Here's the drawing with two shaded views (mm, measured from the low corner). I have some questions. A direction names the side the tool comes from. Round coordinates to 2 decimals unless told otherwise and drop trailing zeros. Write each loop counter-clockwise with the first axis right and the second up, starting at its lowest first coordinate (ties: lowest second). Pieces come first, ordered by that corner, then holes. Notation, with made-up numbers: M -15,-7.75 L 39,-7.75 A33 ccw 39,24.25 Z; hole C 6,43 d4. An arc over 180 degrees is marked long. Answer as a JSON object with one key per item and string values. Group by question number.
1) If we mould it in two halves opening along Z, with no side actions, what happens to the marked faces 3, 4 and 5? For each: +Z half, -Z half, draft (parallel to the pull), parting line (faces both ways), or undercut.
2) On a 3-axis mill with a long thin cutter (end or side, diameter ignored), from which of +Z, -Z, +X, -X, +Y, -Y can I reach the whole of each face in a straight line? I mean the marked faces 1 and 2. Say none if no direction works.
3) I'm going to push flat-ended pins straight in: pin 1 Ø5 at (y, z) = (20.5, 49.5) entering from +X; pin 2 Ø3 at (y, z) = (24.5, 70) entering from -X; pin 3 Ø5 at (x, y) = (79, 24) entering from +Z; pin 4 Ø3 at (x, y) = (111.5, 23) entering from -Z. Where does each tip first touch, or does it pass through?
4) Suppose I cut it at B-B, the plane z = 58. Write out the boundary of the cut face in (x, y), and give its area (3 significant figures).
5) Please list where these lines run through material, in increasing order: L1, parallel to X at y = 27, z = 58; L2, parallel to Z at x = 142, y = 17; L3, parallel to Y at x = 118.5, z = 93. Write a range as [from, to].
6) Suppose I cut it at A-A, the plane x = 113. Write out the boundary of the cut face in (y, z).
7) Suppose I cut it at C-C, the plane x = 90.5. Write out the boundary of the cut face in (y, z), and give its area (3 significant figures).
8) Suppose I cut it at D-D, the plane z = 30. Write out the boundary of the cut face in (x, y), and give its area (3 significant figures).
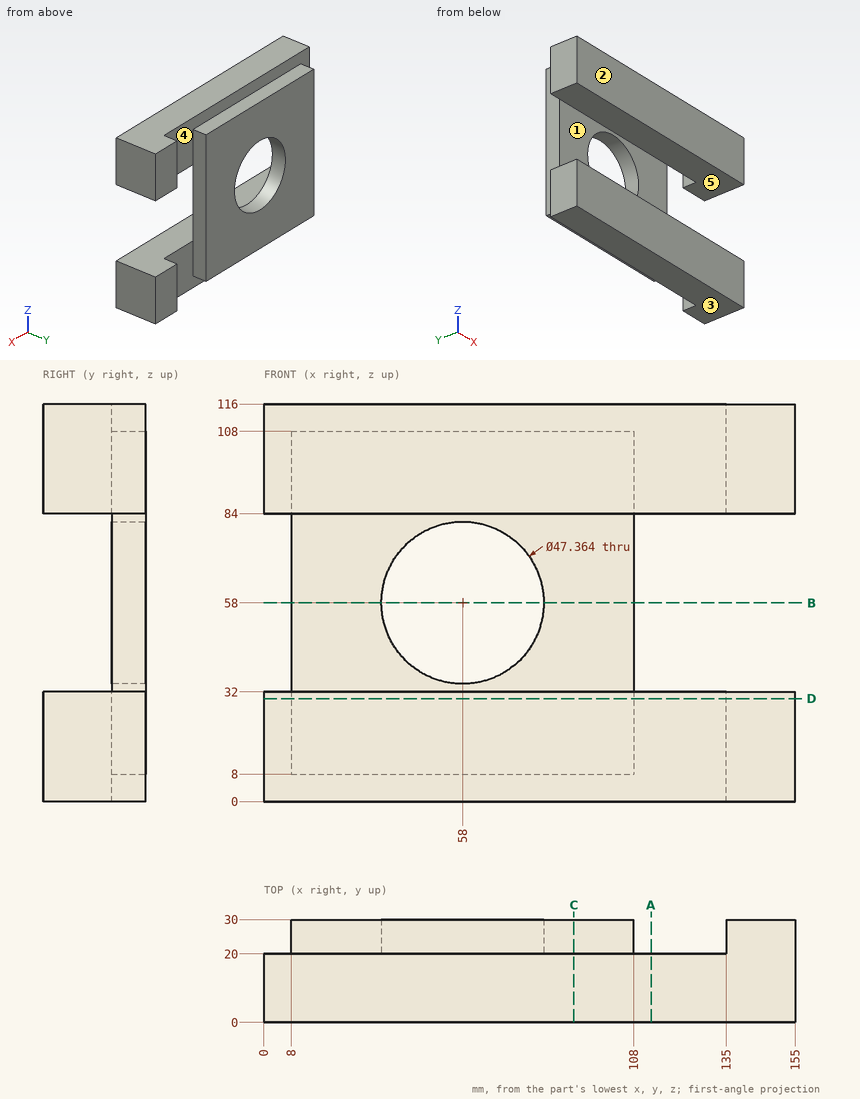
Results:
{
 "1": {"face 3": "-Z half", "face 4": "draft", "face 5": "undercut"},
 "2": {"face 1": "+X, -X, -Y", "face 2": "+Z, -Z, +X, -X, -Y"},
 "3": {"pin 1": "x = 108", "pin 2": "x = 8", "pin 3": "z = 108", "pin 4": "through"},
 "4": {"outline": "M 8,20 L 34.32,20 L 34.32,30 L 8,30 Z; M 81.68,20 L 108,20 L 108,30 L 81.68,30 Z", "area": "526 mm^2"},
 "5": {"L1": "[8, 34.32], [81.68, 108]", "L2": "[0, 32], [84, 116]", "L3": "[0, 20]"},
 "6": {"outline": "M 0,0 L 20,0 L 20,32 L 0,32 Z; M 0,84 L 20,84 L 20,116 L 0,116 Z"},
 "7": {"outline": "M 0,0 L 20,0 L 20,8 L 30,8 L 30,108 L 20,108 L 20,116 L 0,116 L 0,84 L 20,84 L 20,32 L 0,32 Z", "area": "2,280 mm^2"},
 "8": {"outline": "M 0,0 L 155,0 L 155,30 L 135,30 L 135,20 L 108,20 L 108,30 L 8,30 L 8,20 L 0,20 Z", "area": "4,300 mm^2"}
}
